Print and shaded views of the part. All mm, measured from the part's lowest x, y and z. A direction names the side the tool comes from. Give positions to 0.01 mm unless a question says otherwise; leave off trailing zeros. Loops run counter-clockwise (first coordinate to the right, second up) from the corner with the lowest first, then second, coordinate; pieces in that order, holes last. Notation, with made-up numbers: M -3.5,-37.5 L 9.5,-37.5 A25 cw 9.5,-19.5 Z; hole C 62,-19.75 d5. An arc over 180 degrees is marked long. Answer as CSV lines item,"result".
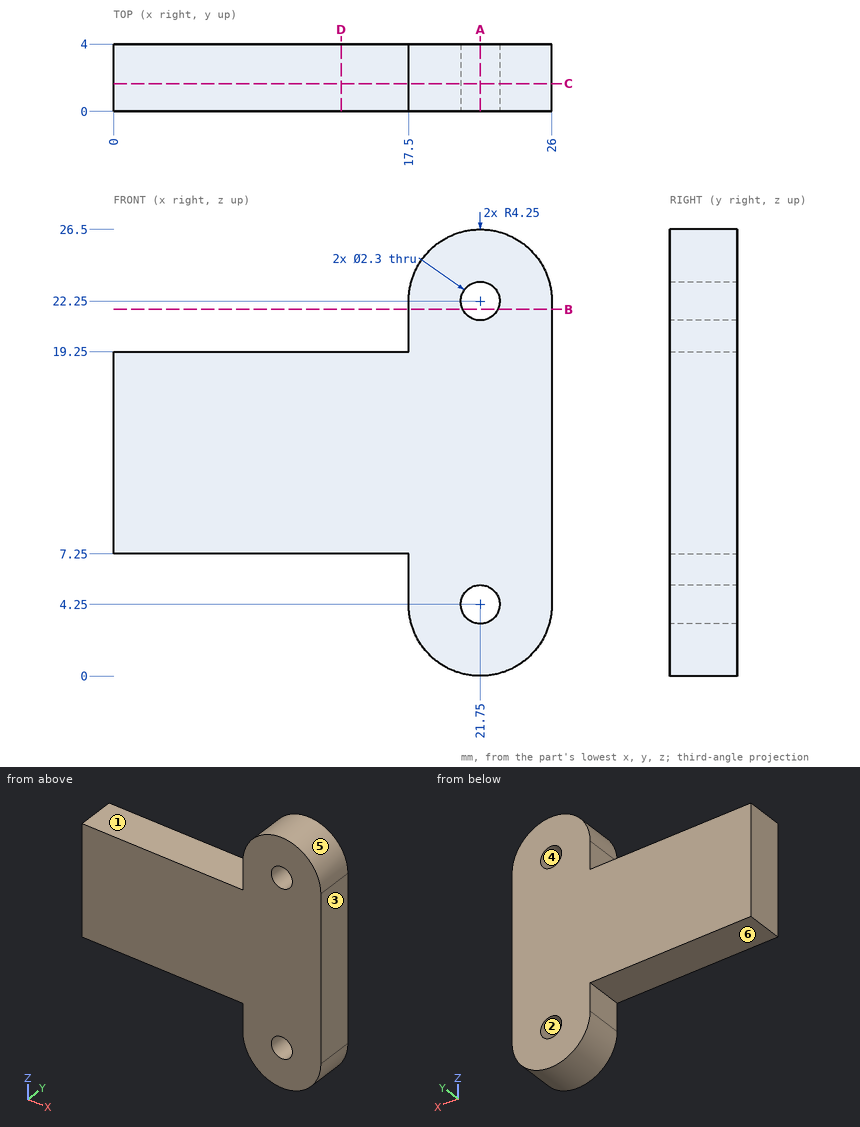
Q1. Cut at D-D (x = 13.5). Write the cut outline in (y, z).
Solution:
outline,"M 0,7.25 L 4,7.25 L 4,19.25 L 0,19.25 Z"
Q2. Mould opens along Z. For the marked faces 1, 2, 3 and 4 say: released by +Z, released by -Z, zero draft, split by the parting line, or undercut.
Solution:
face 1,"released by +Z"
face 2,"undercut"
face 3,"zero draft"
face 4,"undercut"
Q3. Cut at C-C (y = 1.65). Write the cut outline in (x, z).
Solution:
outline,"M 0,7.25 L 17.5,7.25 L 17.5,4.25 A4.25 ccw 26,4.25 L 26,22.25 A4.25 ccw 17.5,22.25 L 17.5,19.25 L 0,19.25 Z; hole C 21.75,4.25 d2.3; hole C 21.75,22.25 d2.3"
Q4. Wall check: line 1 (X direction, y = 1.1, z = 22.25); line 2 (Z direction, x = 21.25, y = 3.6); line 3 (Z direction, x = 9.5, y = 3.7). Give the ranges that are in metal, low to high. Write a range as [from, to].
Solution:
line 1,"x = [17.5, 20.6], [22.9, 26]"
line 2,"z = [0.03, 3.21], [5.29, 21.21], [23.29, 26.47]"
line 3,"z = [7.25, 19.25]"
Q5. Pin check, flat tips, straight feed: P1, Ø2, axis at x = 8.5, y = 1.5, coming from the -Z side; P2, Ø10, axis at x = 11.5, z = 13, coming from the -Y side; P3, Ø2, axis at x = 10.5, y = 1.5, coming from the +Z side; P4, Ø0.9, axis at y = 3, z = 5, coming from the -X side. Stop position of each tip, or through.
Solution:
P1,"stops at z = 7.25"
P2,"stops at y = 0"
P3,"stops at z = 19.25"
P4,"stops at x = 17.5"
Q6. Cut at B-B (z = 21.75). Write the cut outline in (x, y), and give its area (3 significant figures).
Solution:
outline,"M 17.5,0 L 20.71,0 L 20.71,4 L 17.5,4 Z; M 22.79,0 L 26,0 L 26,4 L 22.79,4 Z"
area,"25.7 mm²"
Q7. Which spindle directions (+Z, -Z, +X, -X, +Y, -Y) get a long thin tool onto all of the face, cutting with end or side? Do the marked faces 5 and 6. Say none if no direction does.
Solution:
face 5,"+Z, +Y, -Y"
face 6,"-Z, -X, +Y, -Y"
Q8. Cut at A-A (x = 21.75). Write the cut outline in (y, z), and give its area (3 significant figures).
Solution:
outline,"M 0,0 L 4,0 L 4,3.1 L 0,3.1 Z; M 0,5.4 L 4,5.4 L 4,21.1 L 0,21.1 Z; M 0,23.4 L 4,23.4 L 4,26.5 L 0,26.5 Z"
area,"87.6 mm²"
